Geometry: final body of the model. Coordinates: model frame, mm. Give positions to 0.01 mm unless a question says otherwise; leave off trailing zeros. Write each loop counter-clockwise with the first axis right and the second up, starting at its lowest first coordinate (ties: lowest second). Pieces come first, ordered by that corner, then holes.
Autodesk Inventor part; units mm, degrees
ref_plane "YZ Plane" through (0, 0, 0) normal (1, 0, 0) x (0, 1, 0)
ref_plane "XZ Plane" through (0, 0, 0) normal (0, 1, 0) x (-1, 0, 0)
ref_plane "XY Plane" through (0, 0, 0) normal (0, 0, 1) x (1, 0, 0)
sketch "Esboço1" plane through (0, 0, 0) normal (0, 1, 0) x (-1, 0, 0)
  line L0 (-18.5, 20) -> (18.5, 20)
  line L1 (20, 18.5) -> (20, -18.5)
  line L2 (18.5, -20) -> (-18.5, -20)
  line L3 (-20, -18.5) -> (-20, 18.5)
  line L4 (-20, 20) -> (20, -20) construction
  line L5 (20, 20) -> (-20, -20) construction
  line L6 (-18.5, -18.5) -> (18.5, -18.5)
  line L7 (18.5, -18.5) -> (18.5, 18.5)
  line L8 (18.5, 18.5) -> (-18.5, 18.5)
  line L9 (-18.5, 18.5) -> (-18.5, -18.5)
  line L10 (-18.5, -18.5) -> (18.5, 18.5) construction
  line L11 (18.5, -18.5) -> (-18.5, 18.5) construction
  arc A0 (20, 18.5) -> (18.5, 20) centre (18.5, 18.5) ccw
  arc A1 (-18.5, 20) -> (-20, 18.5) centre (-18.5, 18.5) ccw
  arc A2 (-20, -18.5) -> (-18.5, -20) centre (-18.5, -18.5) ccw
  arc A3 (18.5, -20) -> (20, -18.5) centre (18.5, -18.5) ccw
  point P0 (0, 0)
  dimension "d0" = 40
  dimension "d1" = 40
  dimension "d2" = 1.5
  dimension "d3" = 1.5
extrude "Extrusão1" add sketch "Esboço1" along normal mid plane 2500
equation "\"d3\" = d2"
properties part number "MSI-102" material "Aço inoxidável AISI 304"
Item 1: Line query: L1, parallel to X at y = -217, z = -7. Output: solid intervals per line, ascending.
Found:
L1: x = -20 to -18.5, 18.5 to 20
Item 2: Section C-C, the plane z = -3. Return the cut outline in (x, y), plus the area to 3 significant figures.
Found:
outline: (-20, -1250) - (-18.5, -1250) - (-18.5, 1250) - (-20, 1250) - close; (18.5, -1250) - (20, -1250) - (20, 1250) - (18.5, 1250) - close
area: 7,500 mm2
Item 3: Section B-B, the plane y = -892. Return the cut outline in (x, z), plus the area to 3 significant figures.
Found:
outline: (-20, -18.5) arc R1.5 ccw to (-18.5, -20) - (18.5, -20) arc R1.5 ccw to (20, -18.5) - (20, 18.5) arc R1.5 ccw to (18.5, 20) - (-18.5, 20) arc R1.5 ccw to (-20, 18.5) - close; hole (-18.5, -18.5) - (18.5, -18.5) - (18.5, 18.5) - (-18.5, 18.5) - close
area: 229 mm2
Item 4: Section A-A, the plane x = -9.5. Return the cut outline in (y, z).
Found:
outline: (-1250, -20) - (1250, -20) - (1250, -18.5) - (-1250, -18.5) - close; (-1250, 18.5) - (1250, 18.5) - (1250, 20) - (-1250, 20) - close
